Input: part model. Units: mm. Frame: model coordinates. Face numbers are marked on the shaded views. A direction names the side the tool comes from. Coordinates: 2 decimals unless noted, no trailing zeros. Order: outer loops, then holes, each group sorted by start corner. A loop starts at its lowest first (then second) coordinate and runs counter-clockwise, first axis right, second up. Notation, with made-up numbers: (69.25, -4.5) -> (76.25, -4.5) arc R5 cw to (76.25, 4.5) -> close; hole circle Ø9 at (17, 43). An arc over 180 degrees is marked (long way). Answer as CSV lines item,"result".
Autodesk Inventor part; units mm, degrees
ref_plane "YZ Plane" through (0, 0, 0) normal (1, 0, 0) x (0, 1, 0)
ref_plane "XZ Plane" through (0, 0, 0) normal (0, 1, 0) x (-1, 0, 0)
ref_plane "XY Plane" through (0, 0, 0) normal (0, 0, 1) x (1, 0, 0)
sketch "Sketch1" plane through (0, 0, 0) normal (0, 0, 1) x (1, 0, 0)
  line L0 (0, 0.8293) -> (0, 13.3857)
  line L1 (2.5, 0) -> (2.5, 14)
  line L2 (2.5, 14) -> (3.5, 14)
  line L3 (3.5, 14) -> (3.5, 4)
  line L4 (3.5, 4) -> (5, 4)
  line L5 (5, 4) -> (5, 0)
  line L6 (5, 0) -> (2.5, 0)
  point P0 (0, 0)
  dimension "d0" = 2.5
  dimension "d2" = 3.5
  dimension "d3" = 10
  dimension "d4" = 4
  dimension "d5" = 5
revolve "Revolution1" add sketch "Sketch1" angle 360 about axis through (0, 0.8293, 0) along (0, 1, 0)
sketch "Sketch2" plane through (0, 0, 0) normal (0, 0, 1) x (1, 0, 0)
  circle A0 centre (0, 2) radius 1.5
  point P0 (0, 0)
  dimension "d7" = 2
  dimension "d8" = 3
extrude "Extrusion1" cut sketch "Sketch2" against normal blind 10
thread "Thread1"
sketch "Sketch3" plane through (0, 14, 0) normal (0, 1, 0) x (1, 0, 0)
  circle A0 centre (0, 0) radius 3.5
  circle A1 centre (0, 3.8726) radius 0.7037
  circle A2 centre (-1.399, 3.6111) radius 0.7037
  circle A3 centre (-2.609, 2.8619) radius 0.7037
  circle A4 centre (-3.4666, 1.7262) radius 0.7037
  circle A5 centre (-3.8561, 0.3573) radius 0.7037
  circle A6 centre (-3.7248, -1.0598) radius 0.7037
  circle A7 centre (-3.0904, -2.3338) radius 0.7037
  circle A8 centre (-2.0387, -3.2926) radius 0.7037
  circle A9 centre (-0.7116, -3.8067) radius 0.7037
  circle A10 centre (0.7116, -3.8067) radius 0.7037
  circle A11 centre (2.0387, -3.2926) radius 0.7037
  circle A12 centre (3.0904, -2.3338) radius 0.7037
  circle A13 centre (3.7248, -1.0598) radius 0.7037
  circle A14 centre (3.8561, 0.3573) radius 0.7037
  circle A15 centre (3.4666, 1.7262) radius 0.7037
  circle A16 centre (2.609, 2.8619) radius 0.7037
  circle A17 centre (1.399, 3.6111) radius 0.7037
  dimension "d15" = 360
extrude "Extrusion2" cut sketch "Sketch3" against normal blind 10 contours A0 A14 | A0 A14 | A15 A0 | A0 A15 | A13 A0 | A0 A13 | A16 A0 | A0 A16 | A12 A0 | A0 A12 | A17 A0 | A0 A17 | A11 A0 | A0 A11 | A1 A0 | A0 A1 | A10 A0 | A0 A10 | A2 A0 | A0 A2 | A9 A0 | A0 A9 | A3 A0 | A0 A3 | A8 A0 | A0 A8 | A4 A0 | A0 A4 | A7 A0 | A0 A7 | A5 A0 | A0 A5 | A6 A0 | A0 A6
properties part number "exBolt"
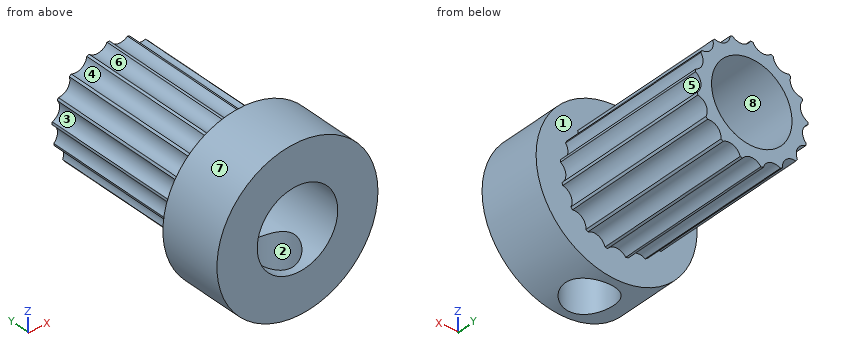
1. Cut plane C-C (y = 2.5). Return the cut outline in (x, z), plus the area to 3 significant figures.
Findings:
outline,"(-1.41, -4.8) -> (-1.41, -2.06) arc R2.5 cw (long way) to (1.41, -2.06) -> (1.41, -4.8) arc R5 ccw (long way) to start"
area,"51.6 mm2"
2. Cut plane D-D (z = 4.25). Return the cut outline in (x, y).
Findings:
outline,"(-2.63, 0) -> (2.63, 0) -> (2.63, 4) -> (-2.63, 4) -> close"
3. Contact query for flat-ended pins moving along their axis: pin 1 (5 mm diameter, centred on x = 2.5, y = 8, fed in from +Z); pin 2 (3 mm diameter, centred on x = 0, y = 7.5, fed in from -Z); pin 3 (2.5 mm diameter, centred on x = 0, y = 2, fed in from -Z). Output: stop coordinate, or through.
Findings:
pin 1,"stops at z = 3.5"
pin 2,"stops at z = -3.45"
pin 3,"stops at z = 2.17"
4. Cut plane A-A (z = -0.5). Return the cut outline in (x, y), plus the area to 3 significant figures.
Findings:
outline,"(-4.97, 0) -> (-2.45, 0) -> (-2.45, 14) -> (-3.17, 14) -> (-3.17, 4) -> (-4.97, 4) -> close; (2.45, 0) -> (4.97, 0) -> (4.97, 4) -> (3.17, 4) -> (3.17, 14) -> (2.45, 14) -> close"
area,"34.6 mm2"
5. Mould query, pull axis Z, two halves, no side actions, for the marked faces 6, 7 and 8. Classes: released by +Z, released by -Z, zero draft, split by the parting line, or undercut.
Findings:
face 6,"released by +Z"
face 7,"split by the parting line"
face 8,"undercut"
6. Cut plane B-B (x = -1). Return the cut outline in (y, z), plus the area to 3 significant figures.
Findings:
outline,"(0, -4.9) -> (0.88, -4.9) -> (0.88, -2.29) -> (0, -2.29) -> close; (0, 2.29) -> (14, 2.29) -> (14, 3.16) -> (4, 3.16) -> (4, 4.9) -> (0, 4.9) -> close; (3.12, -4.9) -> (4, -4.9) -> (4, -3.03) -> (14, -3.03) -> (14, -2.29) -> (3.12, -2.29) -> close"
area,"31.2 mm2"
7. Reachability of the marked faces 1, 2, 3, 4 and 5 from +Z, -Z, +X, -X, +Y, -Y: full face, straight path, thin tool, end or side. Return the list, or none.
Findings:
face 1,"+Y"
face 2,"-Z"
face 3,"-X, +Y"
face 4,"+Z, +Y"
face 5,"+X, +Y"
8. Ray query, line 1 along Z through (x, y) = (0, 5); line 2 along Y through (x, z) = (0, -3.1); line 3 along Y through (x, z) = (0, -3.95). Return the intervals inside material, ascending.
Findings:
line 1,"z = -3.17 to -2.5, 2.5 to 3.5"
line 2,"y = 0 to 0.5, 3.5 to 14"
line 3,"y = 0 to 0.5, 3.5 to 4"
